Autodesk Inventor part; units mm, degrees
ref_plane "YZ Plane" through (0, 0, 0) normal (1, 0, 0) x (0, 1, 0)
ref_plane "XZ Plane" through (0, 0, 0) normal (0, 1, 0) x (-1, 0, 0)
ref_plane "XY Plane" through (0, 0, 0) normal (0, 0, 1) x (1, 0, 0)
sketch "Sketch1" plane through (0, 0, 0) normal (0, 0, 1) x (1, 0, 0)
  circle A0 centre (0, 0) radius 11.125
  circle A1 centre (0, 0) radius 12.875
  circle A2 centre (0, 0) radius 17.875
  dimension "d0" = 22.25
  dimension "d1" = 25.75
  dimension "d2" = 5
extrude "Extrusion1" add sketch "Sketch1" along normal blind 5 contours A0 | A1 | A2
extrude "Extrusion2" add sketch "Sketch1" along normal blind 5.5 from surface at 5 contours A0 | A1
extrude "Extrusion3" add sketch "Sketch1" along normal blind 2.5 from surface at 10.5 contours A0
fillet "Fillet1" radius 1.25 1 edges at (-17.875, 0, 0)
sketch "Sketch2" plane through (0, 0, 0) normal (0, 0, -1) x (-1, 0, 0)
  line L0 (-12.5, -12.5) -> (12.5, -12.5)
  line L1 (12.5, -12.5) -> (12.5, 12.5)
  line L2 (12.5, 12.5) -> (-12.5, 12.5)
  line L3 (-12.5, 12.5) -> (-12.5, -12.5)
  line L4 (-12.5, -12.5) -> (12.5, 12.5) construction
  line L5 (12.5, -12.5) -> (-12.5, 12.5) construction
  line L6 (-12.5, 12.5) -> (12.5, 12.5) construction
  line L7 (12.5, 12.5) -> (12.5, -12.5) construction
  line L8 (12.5, -12.5) -> (-12.5, -12.5) construction
  line L9 (-12.5, -12.5) -> (-12.5, 12.5) construction
  line L10 (3.8655, -10) -> (-3.8817, -10)
  line L11 (-3.8817, -10) -> (-3.8817, -7.9579)
  line L12 (-3.8817, -7.9579) -> (-1.3371, -7.9579)
  line L13 (-1.3371, -7.9579) -> (-1.3371, 7.9579)
  line L14 (-1.3371, 7.9579) -> (-3.8817, 7.9579)
  line L15 (-3.8817, 7.9579) -> (-3.8817, 10)
  line L16 (-3.8817, 10) -> (3.8655, 10)
  line L17 (3.8655, 10) -> (3.8655, 7.9579)
  line L18 (3.8655, 7.9579) -> (1.3209, 7.9579)
  line L19 (1.3209, 7.9579) -> (1.3209, -7.9579)
  line L20 (1.3209, -7.9579) -> (3.8655, -7.9579)
  line L21 (3.8655, -7.9579) -> (3.8655, -10)
  point P0 (0, 0)
  dimension "d10" = 25
  dimension "d11" = 25
extrude "Extrusion4" cut sketch "Sketch2" against normal blind 0.25 contours L10 L11 L12 L13 L14 L15 L16 L17 L18 L19 L20 L21
chamfer "Chamfer1" distance 0.25 angle 45 12 edges at (0.0081, -10, 0.25) (3.8817, -8.9789, 0.25) (2.6094, -7.9579, 0.25) (1.3371, 0, 0.25) (2.6094, 7.9579, 0.25) (3.8817, 8.9789, 0.25) (0.0081, 10, 0.25) (-3.8655, 8.9789, 0.25) (-2.5932, 7.9579, 0.25) (-1.3209, 0, 0.25) (-2.5932, -7.9579, 0.25) (-3.8655, -8.9789, 0.25)
properties part number "Inner Ring Press"
Can you work these out from the model? Positions are in its coordinate system, mm. A direction names the side the tool comes from. Coordinates: 2 decimals unless noted, no trailing zeros. Write each loop counter-clockwise with the first axis right and the second up, starting at its lowest first coordinate (ties: lowest second). Pieces come first, ordered by that corner, then holes. Notation, with made-up numbers: (71, -38) - (107, -38) arc R28 cw to (107, -16) - close; hole circle Ø11 at (-39.75, -39.5). An arc over 180 degrees is marked (long way). Return JSON: item names as keys, results as strings.
Q1. Please list where these lines run through material, in increasing order: L1, parallel to Y at x = 7.5, z = 11.5; L2, parallel to Z at x = 11.5, y = 4; L3, parallel to Z at x = 2, y = -9.5. Write a range as from..to.
Computed values:
{"L1": "y = -8.22..8.22", "L2": "z = 0..10.5", "L3": "z = 0.25..13"}
Q2. Thinking about a two-plate mould opening in X: for faces 3 (the flat face through (3, 0, 0)), 4 (the flat face through (0, 0, 0.25)), 5 (the cylindrical face through (-2.79, 12.57, 7.71)), which applies, +X half, -X half, draft (parallel to the pull), parting line (faces both ways), or undercut?
Computed values:
{"face 3": "draft", "face 4": "undercut", "face 5": "parting line"}
Q3. If we section it at D-D (z = 8.5): Please give me the cut outline in (x, y) (3 decimals).
Computed values:
{"outline": "circle Ø25.75 at (0, 0)"}
Q4. I'm going to push flat-ended pins straight in: pin 1 Ø1 at (y, z) = (9, 11.5) entering from -X; pin 2 Ø5 at (x, z) = (6.5, 9.5) entering from -Y; pin 3 Ø6 at (y, z) = (8.5, 11) entering from -X. Where does each tip first touch, or does it pass through?
Computed values:
{"pin 1": "stops at x = -7.18", "pin 2": "stops at y = -12.24", "pin 3": "stops at x = -11.62"}
Q5. On a 3-axis mill with a long thin cutter (end or side, diameter ignored), from which of +Z, -Z, +X, -X, +Y, -Y can I reach the whole of each face in a straight line? I mean faces 1 (the flat face through (0, 0, 13)), 2 (the flat face through (8, -12, 5)). Say none if no direction works.
Computed values:
{"face 1": "+Z, +X, -X, +Y, -Y", "face 2": "+Z"}
Q6. If we section it at C-C (z = 2.5): Please give me the cut outline in (x, y) (3 decimals), then the cut area to 3 significant figures.
Computed values:
{"outline": "circle Ø35.75 at (0, 0)", "area": "1,000 mm2"}
